Read the model definition and answer for the solid it produces. Units are mm, in the model's axes. Face numbers are marked on the shaded views. A direction names the side the tool comes from. Give positions to 0.01 mm unless a question says otherwise; leave off trailing zeros. Order: outer loops, then holes, each group sorted by start corner. A loop starts at its lowest first (then second) coordinate and runs counter-clockwise, first axis right, second up. Notation, with made-up numbers: (42, -35.5) - (50, -35.5) arc R31 cw to (50, -5.5) - close; hole circle Ø1 at (17, 17). An arc over 180 degrees is marked (long way). Use a Markdown table: item, result. Add a question column.
1. A cutting plane is placed at A-A on z = 7. Determine the outline of the cut face in (x, y).
2. For a pull along Y with two mould halves and no side action, classify the marked faces 3, 4, 5 and 6 as released by +Y, released by -Y, zero draft, split by the parting line, or undercut.
3. A cutting plane is placed at D-D on z = 21. Determine the outline of the cut face in (x, y).
4. Which of the six approach directions +Z, -Z, +X, -X, +Y, -Y give full straight-line access (tool end or side, diameter ignored) to the marked faces 1 and 2?
5. Consider L1, parallel to Y at x = 20.25, z = 10; L2, parallel to Z at x = 2, y = 2; L3, parallel to Y at x = 3, z = 21.25. Determine where each line is inside the solid, lowest interval first.
6. A cutting plane is placed at C-C on y = 2.15. Determine the outline of the cut face in (x, z).
7. A cutting plane is placed at B-B on x = 3.25. Determine the outline of the cut face in (y, z).
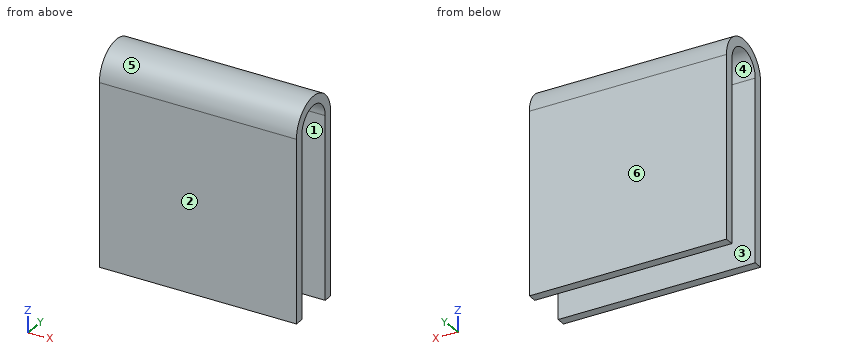
```python
from build123d import *

# Parameters (mm, degrees)
TABAN_FLAN_1_DEPTH = 21.5


# Sheet-metal steps are written as plain solids
with BuildPart() as part:
    # Çizim1 → Taban-Flanş1 (new body)
    with BuildSketch(Plane.YZ):
        with BuildLine():
            Line((0, 0), (0, 19.85))
            ThreePointArc((0, 19.85), (2.15, 22), (4.3, 19.85))
            Line((4.3, 19.85), (4.3, 0))
            Line((4.3, 0), (5.3, 0))
            Line((5.3, 0), (5.3, 19.85))
            ThreePointArc((5.3, 19.85), (2.15, 23), (-1, 19.85))
            Line((-1, 19.85), (-1, 0))
            Line((-1, 0), (0, 0))
        make_face()
    extrude(amount=TABAN_FLAN_1_DEPTH)


solid = part.part
```
Output values:
| question | item | result |
|---|---|---|
| 1 | outline | (0, -1) - (21.5, -1) - (21.5, 0) - (0, 0) - close; (0, 4.3) - (21.5, 4.3) - (21.5, 5.3) - (0, 5.3) - close |
| 2 | face 3 | undercut |
| 2 | face 4 | undercut |
| 2 | face 5 | split by the parting line |
| 2 | face 6 | released by +Y |
| 3 | outline | (0, -0.78) - (21.5, -0.78) - (21.5, 0.33) - (0, 0.33) - close; (0, 3.97) - (21.5, 3.97) - (21.5, 5.08) - (0, 5.08) - close |
| 4 | face 1 | -Z, +X, -X |
| 4 | face 2 | +Z, -Z, +X, -X, -Y |
| 5 | L1 | -1 to 0, 4.3 to 5.3 |
| 5 | L2 | 21.99 to 23 |
| 5 | L3 | -0.67 to 0.52, 3.78 to 4.97 |
| 6 | outline | (0, 22) - (21.5, 22) - (21.5, 23) - (0, 23) - close |
| 7 | outline | (-1, 0) - (0, 0) - (0, 19.85) arc R2.15 cw to (4.3, 19.85) - (4.3, 0) - (5.3, 0) - (5.3, 19.85) arc R3.15 ccw to (-1, 19.85) - close |
